The listing builds one solid part. Answer for the finished solid, in the listing's coordinates (mm). Give positions to 0.01 mm unless a question says otherwise; leave off trailing zeros. Order: outer loops, then holes, each group sorted by start corner. A loop starts at its lowest first (then second) coordinate and runs counter-clockwise, first axis right, second up. Notation, with made-up numbers: (-10, 72.25) - (8, 72.25) arc R5 cw to (8, 79.25) - close; hole circle Ø10 at (62, -15.5). An arc over 180 degrees is marked (long way). Answer as a JSON object with one key per item and string values. Group by question number.
Q1. Consider line 1 (Y direction, x = 10, z = 0.85); line 2 (X direction, y = 8.5, z = 0.4); line 3 (Y direction, x = 11, z = 0.8). Determine where each line is inside the solid, lowest interval first.
Q2. A cutting plane is placed at B-B, the plane y = 0. Give the vertices of the cut face in (x, z).
Q3. A cutting plane is placed at C-C, the plane z = 0.75. Give the vertices of the cut face in (x, y).
Q4. The mould has two halves that part along Y. Classify faces 1 (the face through (2.003, 0.631, 0.493)), 2 (the face through (-5, 4.9, 0.5)), 3 (the face through (24.57, 14.55, 0.49)): released by +Y, released by -Y, zero draft, split by the parting line, or undercut.
Q5. A cutting plane is placed at A-A, the plane x = 10. Give the vertices of the cut face in (y, z).
Q6. A cutting plane is placed at D-D, the plane x = 0.5. Give the vertices of the cut face in (y, z).
from build123d import *

# Parameters (mm, degrees)
SKETCH_R  = 2.1
PAD_DEPTH = 1


with BuildPart() as part:
    # Sketch → Pad (new body)
    with BuildSketch(Plane.XY):
        with BuildLine():
            Line((-3.5, 15), (23.5, 15))
            ThreePointArc((25, 13.5), (24.56066, 14.56066), (23.5, 15))
            Line((25, 13.5), (25, -3.5))
            ThreePointArc((23.5, -5), (24.56066, -4.56066), (25, -3.5))
            Line((23.5, -5), (-3.5, -5))
            ThreePointArc((-5, -3.5), (-4.56066, -4.56066), (-3.5, -5))
            Line((-5, -3.5), (-5, 13.5))
            ThreePointArc((-3.5, 15), (-4.56066, 14.56066), (-5, 13.5))
        make_face()
        Circle(SKETCH_R, mode=Mode.SUBTRACT)
        with Locations((0, 10)):
            Circle(SKETCH_R, mode=Mode.SUBTRACT)
        with Locations((10, 0)):
            Circle(SKETCH_R, mode=Mode.SUBTRACT)
        with Locations((20, 0)):
            Circle(SKETCH_R, mode=Mode.SUBTRACT)
        with Locations((10, 10)):
            Circle(SKETCH_R, mode=Mode.SUBTRACT)
        with Locations((20, 10)):
            Circle(SKETCH_R, mode=Mode.SUBTRACT)
    extrude(amount=PAD_DEPTH)


solid = part.part
Reply:
{
 "1": {"line 1": "y = -5 to -2.1, 2.1 to 7.9, 12.1 to 15", "line 2": "x = -5 to -1.47, 1.47 to 8.53, 11.47 to 18.53, 21.47 to 25", "line 3": "y = -5 to -1.85, 1.85 to 8.15, 11.85 to 15"},
 "2": {"outline": "(-5, 0) - (-2.1, 0) - (-2.1, 1) - (-5, 1) - close; (2.1, 0) - (7.9, 0) - (7.9, 1) - (2.1, 1) - close; (12.1, 0) - (17.9, 0) - (17.9, 1) - (12.1, 1) - close; (22.1, 0) - (25, 0) - (25, 1) - (22.1, 1) - close"},
 "3": {"outline": "(-5, -3.5) arc R1.5 ccw to (-3.5, -5) - (23.5, -5) arc R1.5 ccw to (25, -3.5) - (25, 13.5) arc R1.5 ccw to (23.5, 15) - (-3.5, 15) arc R1.5 ccw to (-5, 13.5) - close; hole circle Ø4.2 at (0, 0); hole circle Ø4.2 at (0, 10); hole circle Ø4.2 at (10, 0); hole circle Ø4.2 at (10, 10); hole circle Ø4.2 at (20, 0); hole circle Ø4.2 at (20, 10)"},
 "4": {"face 1": "undercut", "face 2": "zero draft", "face 3": "released by +Y"},
 "5": {"outline": "(-5, 0) - (-2.1, 0) - (-2.1, 1) - (-5, 1) - close; (2.1, 0) - (7.9, 0) - (7.9, 1) - (2.1, 1) - close; (12.1, 0) - (15, 0) - (15, 1) - (12.1, 1) - close"},
 "6": {"outline": "(-5, 0) - (-2.04, 0) - (-2.04, 1) - (-5, 1) - close; (2.04, 0) - (7.96, 0) - (7.96, 1) - (2.04, 1) - close; (12.04, 0) - (15, 0) - (15, 1) - (12.04, 1) - close"}
}
